Input: dimensioned drawing with shaded views. Units: mm. Origin: part minimum x, y, z. A direction names the side the tool comes from. Give positions to 0.01 mm unless a question says otherwise; leave off trailing zeros. Loops run counter-clockwise (first coordinate to the right, second up) from the corner with the lowest first, then second, coordinate; pieces in that order, holes last.
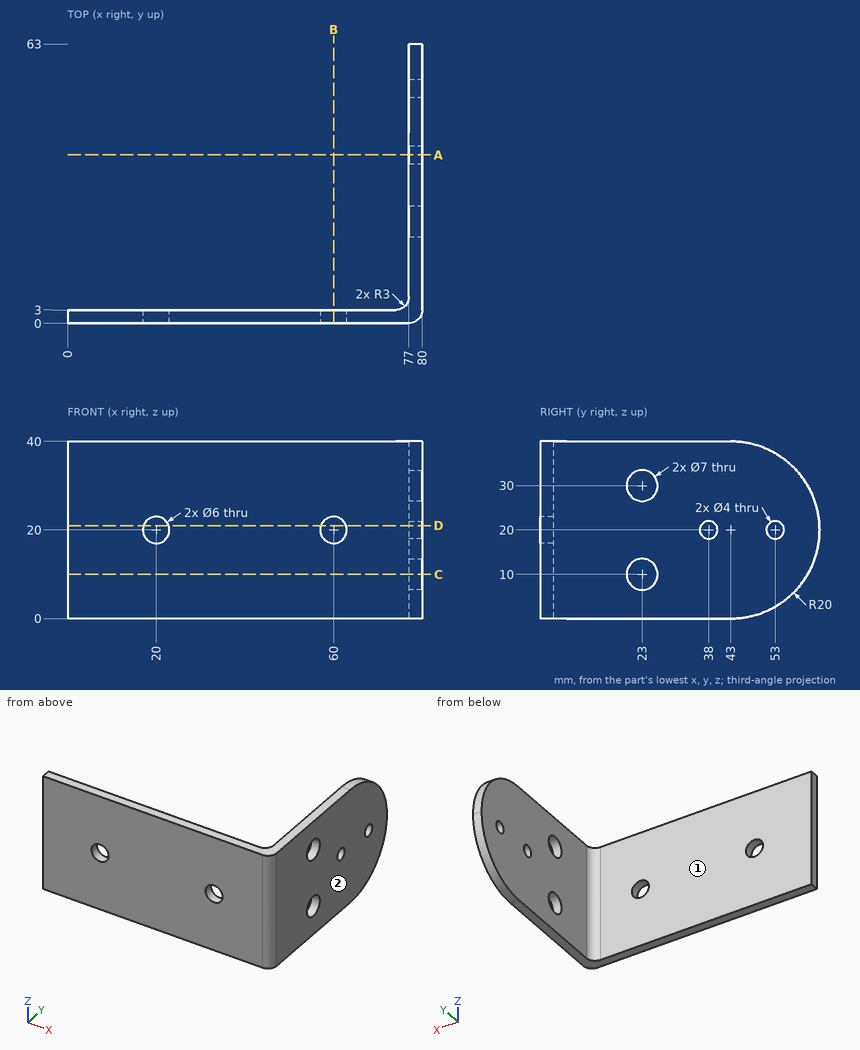
Item 1: Ray query, probe 1 along Y at (x, z) = (78.1, 20); probe 2 along Z at (x, y) = (20, 1.8); probe 3 along Y at (x, z) = (34.5, 27). Return the intervals inside material, ascending.
Values follow:
probe 1: y = 0.21 to 36, 40 to 51, 55 to 63
probe 2: z = 0 to 17, 23 to 40
probe 3: y = 0 to 3
Item 2: Section query A-A on y = 38. Return loops of the section in (x, z), plus the area to 3 significant figures.
Values follow:
outline: (77, 0) - (80, 0) - (80, 18) - (77, 18) - close; (77, 22) - (80, 22) - (80, 40) - (77, 40) - close
area: 108 mm2
Item 3: Section query C-C on z = 10. Return loops of the section in (x, y).
Values follow:
outline: (0, 0) - (77, 0) arc R3 ccw to (80, 3) - (80, 19.5) - (77, 19.5) - (77, 6) arc R3 cw to (74, 3) - (0, 3) - close; (77, 26.5) - (80, 26.5) - (80, 60.32) - (77, 60.32) - close
Item 4: Section query D-D on z = 21. Return loops of the section in (x, y), plus the area to 3 significant figures.
Values follow:
outline: (0, 0) - (17.17, 0) - (17.17, 3) - (0, 3) - close; (22.83, 0) - (57.17, 0) - (57.17, 3) - (22.83, 3) - close; (62.83, 0) - (77, 0) arc R3 ccw to (80, 3) - (80, 36.27) - (77, 36.27) - (77, 6) arc R3 cw to (74, 3) - (62.83, 3) - close; (77, 39.73) - (80, 39.73) - (80, 51.27) - (77, 51.27) - close; (77, 54.73) - (80, 54.73) - (80, 62.97) - (77, 62.97) - close
area: 365 mm2
Item 5: Set-up query: the marked faces 1 and 2. Return all of +Z, -Z, +X, -X, +Y, -Y with unobstructed straight access to the full face (end or side cutting, diameter ignored); none if empty.
Values follow:
face 1: +Z, -Z, -X, +Y
face 2: +Z, -Z, +X, +Y, -Y
Item 6: Section query B-B on x = 60. Return loops of the section in (y, z).
Values follow:
outline: (0, 0) - (3, 0) - (3, 17) - (0, 17) - close; (0, 23) - (3, 23) - (3, 40) - (0, 40) - close
Item 7: Pin query (flat end, axial travel): pin 1 (12 mm diameter, centred on x = 14, z = 26.5, fed in from +Y); pin 2 (9 mm diameter, centred on y = 23, z = 30, fed in from -X); pin 3 (3.5 mm diameter, centred on y = 38, z = 20, fed in from -X). Return the tip coordinate at first contact, or that it passes through.
Values follow:
pin 1: stops at y = 3
pin 2: stops at x = 77
pin 3: passes through
